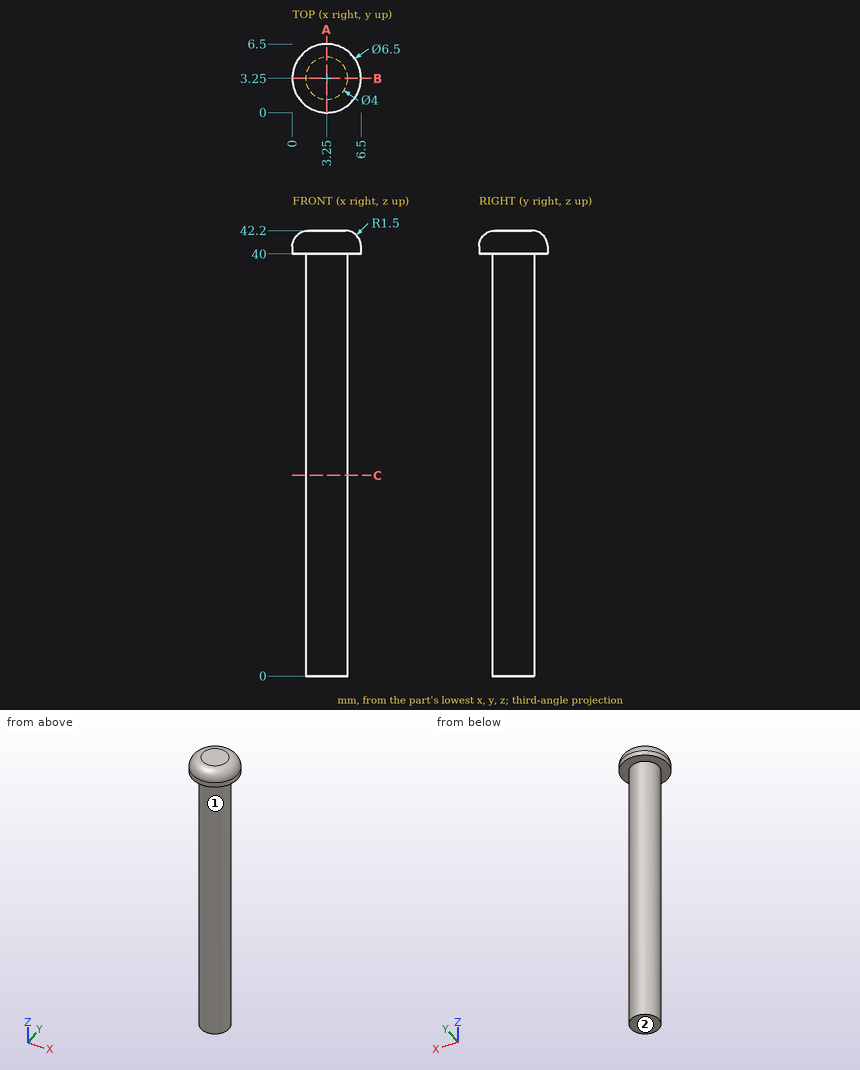
Here's the drawing with two shaded views (mm, measured from the low corner). I have some questions. A direction names the side the tool comes from. Coordinates: 2 decimals unless noted, no trailing zeros. Loops run counter-clockwise (first coordinate to the right, second up) from the corner with the lowest first, then second, coordinate; pieces in that order, holes last. Notation, with made-up numbers: (-33, -20) -> (-23, -20) arc R21 cw to (-23, 18) -> close; hole circle Ø10 at (-21.75, -9). An arc over 180 degrees is marked (long way). Use one line per item in the form item = value. Start each with the question number.
(1) Please list where these lines run through material, in increasing order: line 1 along Y through (x, z) = (3.25, 8); line 2 along Z through (x, y) = (3.25, 6.25); line 3 along Y through (x, z) = (2.5, 11).
(2) If we section it at A-A (x = 3.25): Please give me the cut outline in (y, z), then the cut area to 3 significant figures.
(3) If we section it at C-C (z = 19): Please give me the cut outline in (x, y), then the cut area to 3 significant figures.
(4) Will these pins go through, and if not, where does the flat tip stop? pin 1 (2 mm diameter, centred on y = 1, z = 8.5, fed in from -X); pin 2 (1.5 mm diameter, centred on x = 4.5, z = 8, fed in from +Y); pin 3 (2 mm diameter, centred on y = 5.5, z = 15, fed in from +X).
(5) On a 3-axis mill with a long thin cutter (end or side, diameter ignored), from which of +Z, -Z, +X, -X, +Y, -Y can I reach the whole of each face in a straight line? I mean the marked faces 1 and 2. Say none if no direction works.
Verdict:
q1.line_1 = 1.25 to 5.25
q1.line_2 = 40 to 41.53
q1.line_3 = 1.4 to 5.1
q2.outline = (0, 40) -> (1.25, 40) -> (1.25, 0) -> (5.25, 0) -> (5.25, 40) -> (6.5, 40) -> (6.5, 40.7) arc R1.5 ccw to (5, 42.2) -> (1.5, 42.2) arc R1.5 ccw to (0, 40.7) -> close
q2.area = 173 mm²
q3.outline = circle Ø4 at (3.25, 3.25)
q3.area = 12.6 mm²
q4.pin_1 = 1.69
q4.pin_2 = 5.19
q4.pin_3 = 4.81
q5.face_1 = -Z
q5.face_2 = -Z, +X, -X, +Y, -Y
